Model file for the job. Use its own axes, mm. A direction names the side the tool comes from. Round coordinates to 2 decimals unless told otherwise and drop trailing zeros. Write each loop counter-clockwise with the first axis right and the second up, starting at its lowest first coordinate (ties: lowest second). Pieces come first, ordered by that corner, then holes.
```python
from build123d import *

# Parameters (mm, degrees)
EXTRUDE1_DEPTH     = 17.78
SKETCH3_R          = 1.5875
CUT_EXTRUDE1_DEPTH = 17.78
SKETCH4_W          = 17.78
SKETCH4_H          = 260.35
SKETCH4_H_2        = 189.179603175
SKETCH4_W_2        = 146.050000002
SKETCH4_H_3        = 17.780000002
CUT_EXTRUDE2_DEPTH = 5.08
SKETCH6_R          = 3.302
CUT_EXTRUDE3_DEPTH = 5.08


with BuildPart() as part:
    # Sketch2 → Extrude1 (new body)
    with BuildSketch(Plane.XY):
        Polygon((857.25, -5502.275), (857.25, -5314.95), (157.1625, -5314.95), (157.1625, -5575.3), align=None)
    extrude(amount=-EXTRUDE1_DEPTH)

    # Sketch3 → Cut-Extrude1 (cut)
    with BuildSketch(Plane.XY):
        with Locations((166.0525, -5531.135582009)):
            Circle(SKETCH3_R)
        with Locations((166.0525, -5444.661349205)):
            Circle(SKETCH3_R)
        with Locations((166.0525, -5358.187116401)):
            Circle(SKETCH3_R)
        with Locations((848.36, -5471.826917991)):
            Circle(SKETCH3_R)
        with Locations((848.36, -5409.076150795)):
            Circle(SKETCH3_R)
        with Locations((848.36, -5346.325383599)):
            Circle(SKETCH3_R)
        with Locations((573.0875, -5417.566)):
            Circle(SKETCH3_R)
        with Locations((522.2875, -5417.566)):
            Circle(SKETCH3_R)
        with Locations((471.4875, -5417.566)):
            Circle(SKETCH3_R)
    extrude(amount=-CUT_EXTRUDE1_DEPTH, mode=Mode.SUBTRACT)

    # Sketch4 → Cut-Extrude2 (cut)
    with BuildSketch(Plane.XY):
        with Locations((166.0525, -5445.125)):
            Rectangle(SKETCH4_W, SKETCH4_H)
        with Locations((848.36, -5409.539801588)):
            Rectangle(SKETCH4_W, SKETCH4_H_2)
        with Locations((522.2875, -5417.566)):
            Rectangle(SKETCH4_W_2, SKETCH4_H_3)
    extrude(amount=-CUT_EXTRUDE2_DEPTH, mode=Mode.SUBTRACT)

    # Sketch6 → Cut-Extrude3 (cut)
    with BuildSketch(Plane.XY):
        with Locations((451.507564029, -5410.921064029)):
            Circle(SKETCH6_R)
        with Locations((451.507564029, -5424.210935971)):
            Circle(SKETCH6_R)
        with Locations((593.067435971, -5424.210935971)):
            Circle(SKETCH6_R)
        with Locations((593.067435971, -5410.921064029)):
            Circle(SKETCH6_R)
    extrude(amount=-CUT_EXTRUDE3_DEPTH, mode=Mode.SUBTRACT)


solid = part.part
```
1) Pull direction X, two halves, no side cores. Call faces 3 (the face through (857.25, -5410, -11)), 4 (the face through (521, -5420, -5.08)), 5 (the face through (164, -5443, -5.08)): released by +X, released by -X, zero draft, split by the parting line, or undercut.
2) Flat gauge pins, fed straight in: pin 1 Ø2.5 at (x, y) = (848.36, -5346.33) entering from -Z; pin 2 Ø2.5 at (y, z) = (-5415.5, -2.5) entering from -X; pin 3 Ø5 at (x, y) = (848.36, -5471.83) entering from +Z; pin 4 Ø1.5 at (x, z) = (516, -9) entering from -Y. Where does each tip first touch, or does it go through?
3) Wall check: probe 1 along Y at (x, z) = (848.36, -13); probe 2 along X at (y, z) = (-5428, -1); probe 3 along X at (y, z) = (-5446, -12.5). Give the ranges that are in metal, low to high.
4) Which spindle directions (+Z, -Z, +X, -X, +Y, -Y) get a long thin tool onto all of the face, cutting with end or side? Do faces 1 (the face through (850, -5408, -5.08)), 2 (the face through (503, -5442, 0)). Say none if no direction does.
5) Cut at A-A on z = -9. Give the number of separate pieces and of enclosed holes in the cut face, and give its area (3 significant figures).
6) Cut at D-D on x = 241. List the corners of the cut face in (y, z), and give its area (3 significant figures).
7) Cut at B-B on x = 502. List the corners of the cut face in (y, z).
8) Cut at C-C on x = 613. List the corners of the cut face in (y, z), and give its area (3 significant figures).
Result sheet:
1. face 3: released by +X
1. face 4: undercut
1. face 5: zero draft
2. pin 1: passes through
2. pin 2: stops at x = 174.94
2. pin 3: stops at z = -5.08
2. pin 4: stops at y = -5537.95
3. probe 1: y = -5503.2 to -5473.41, -5470.24 to -5410.66, -5407.49 to -5347.91, -5344.74 to -5314.95
3. probe 2: x = 174.94 to 839.47
3. probe 3: x = 157.16 to 165.2, 166.91 to 857.25
4. face 1: +Z, +X, +Y, -Y
4. face 2: +Z, +X, -X, +Y, -Y
5. separate pieces: 1
5. enclosed holes: 9
5. area: 157,000 mm2
6. outline: (-5566.56, -17.78) - (-5314.95, -17.78) - (-5314.95, 0) - (-5566.56, 0) - close
6. area: 4,470 mm2
7. outline: (-5539.33, -17.78) - (-5314.95, -17.78) - (-5314.95, 0) - (-5408.68, 0) - (-5408.68, -5.08) - (-5426.46, -5.08) - (-5426.46, 0) - (-5539.33, 0) - close
8. outline: (-5527.75, -17.78) - (-5314.95, -17.78) - (-5314.95, 0) - (-5527.75, 0) - close
8. area: 3,780 mm2
